Build history of the part. All positions in model axes, mm. A direction names the side the tool comes from. Round coordinates to 2 decimals unless told otherwise and drop trailing zeros. Write each loop counter-clockwise with the first axis right and the second up, starting at its lowest first coordinate (ties: lowest second). Pieces come first, ordered by that corner, then holes.
Item 1: Band-saw the part on A-A, the plane y = -8.5. Write the cut outline in (x, z).
Item 2: Wall check: probe 1 along X at (y, z) = (-11, 13.5); probe 2 along Z at (x, y) = (19.5, 15); probe 3 along Y at (x, z) = (9.5, 16). Give the ranges that are in metal, low to high.
Item 3: Band-saw the part on D-D, the plane y = 4.5. Write the cut outline in (x, z).
Item 4: 3-axis set-ups, long thin cutter, end or side, ignore diameter. For faces 1 (the flat face through (25.4, -10, 16)), 2 (the flat face through (-19.05, -13, 16)), 3 (the flat face through (-25.4, -9, 16)), 4 (the flat face through (0, 19.05, 3)): which of +Z, -Z, +X, -X, +Y, -Y reach the whole face in a straight line?
Item 5: Band-saw the part on C-C, the plane z = 23. Write the cut outline in (x, y).
Item 6: Mould opens along X. For faces 5 (the flat face through (0, 0, 16)), 6 (the flat face through (-31.75, 0, 3)), 7 (the flat face through (0, -6.35, 16)) say: +X half, -X half, draft (parallel to the pull), parting line (faces both ways), or undercut.
Item 7: Drop flat-ended pins along their axis: pin 1 Ø1 at (x, y) = (12.5, -9.5) entering from +Z; pin 2 Ø3 at (x, z) = (5.5, 16) entering from -Y; pin 3 Ø4 at (y, z) = (-14, 19.5) entering from +X. Give the stop position or say it passes through.
Item 8: Band-saw the part on B-B, the plane x = 4.5. Write the cut outline in (y, z).
```python
from build123d import *

# Parameters (mm, degrees)
F0_W     = 6.35
F0_H     = 12.7
F0_H_2   = 6.35
F0_W_2   = 38.1
F1_DEPTH = 25.4
F2_DEPTH = 6.35


with BuildPart() as f1:
    # F0 (on Top) → F1 (new body)
    with BuildSketch(Plane.XY):
        with Locations((22.225, -12.7)):
            Rectangle(F0_W, F0_H)
        with Locations((22.225, -3.175)):
            Rectangle(F0_W, F0_H_2)
        with Locations((0, -3.175)):
            Rectangle(F0_W_2, F0_H_2)
        with Locations((-22.225, -3.175)):
            Rectangle(F0_W, F0_H_2)
        with Locations((-22.225, -12.7)):
            Rectangle(F0_W, F0_H)
    extrude(amount=F1_DEPTH)

    # F0 (on Top) → F2 (join)
    with BuildSketch(Plane.XY):
        Polygon((31.75, 19.05), (-31.75, 19.05), (-31.75, -19.05), (-25.4, -19.05), (-25.4, -6.35), (-25.4, 0), (-19.05, 0), (19.05, 0), (25.4, 0), (25.4, -6.35), (25.4, -19.05), (31.75, -19.05), align=None)
        with Locations((-22.225, -12.7)):
            Rectangle(F0_W, F0_H)
        with Locations((22.225, -12.7)):
            Rectangle(F0_W, F0_H)
        with Locations((0, -12.7)):
            Rectangle(F0_W_2, F0_H)
    extrude(amount=F2_DEPTH)


solid = f1.part
```
Results:
1. outline: (-31.75, 0) - (31.75, 0) - (31.75, 6.35) - (25.4, 6.35) - (25.4, 25.4) - (19.05, 25.4) - (19.05, 6.35) - (-19.05, 6.35) - (-19.05, 25.4) - (-25.4, 25.4) - (-25.4, 6.35) - (-31.75, 6.35) - close
2. probe 1: x = -25.4 to -19.05, 19.05 to 25.4
2. probe 2: z = 0 to 6.35
2. probe 3: y = -6.35 to 0
3. outline: (-31.75, 0) - (31.75, 0) - (31.75, 6.35) - (-31.75, 6.35) - close
4. face 1: +Z, +X, +Y, -Y
4. face 2: +Z, -Y
4. face 3: +Z, -X, +Y, -Y
4. face 4: +Z, -Z, +X, -X, +Y
5. outline: (-25.4, -19.05) - (-19.05, -19.05) - (-19.05, -6.35) - (19.05, -6.35) - (19.05, -19.05) - (25.4, -19.05) - (25.4, 0) - (-25.4, 0) - close
6. face 5: draft
6. face 6: -X half
6. face 7: undercut
7. pin 1: stops at z = 6.35
7. pin 2: stops at y = -6.35
7. pin 3: stops at x = 25.4
8. outline: (-19.05, 0) - (19.05, 0) - (19.05, 6.35) - (0, 6.35) - (0, 25.4) - (-6.35, 25.4) - (-6.35, 6.35) - (-19.05, 6.35) - close
